The listing builds one solid part. Answer for the finished solid, in the listing's coordinates (mm). A direction names the side the tool comes from. Give positions to 0.01 mm unless a question says otherwise; leave off trailing zeros. Write each loop counter-clockwise with the first axis right and the second up, starting at its lowest first coordinate (ties: lowest second). Pieces come first, ordered by that corner, then holes.
```python
from build123d import *

# Parameters (mm, degrees)
SKETCH1_W             = 110
SKETCH1_H             = 64
SKETCH1_R             = 2.5
SKETCH1_W_2           = 40
SKETCH1_H_2           = 46
BOSS_EXTRUDE1_DEPTH   = 5
FILLET1_R             = 16
FILLET2_R             = 16
SKETCH2_W             = 50
SKETCH2_H             = 5
SKETCH2_W_2           = 20
BOSS_EXTRUDE2_DEPTH   = 46
BOSS_EXTRUDE3_START   = 51
SKETCH1_2_W           = 110
SKETCH1_2_H           = 64
SKETCH1_2_R           = 2.5
SKETCH1_2_W_2         = 40
SKETCH1_2_H_2         = 46
BOSS_EXTRUDE3_DEPTH   = 69
FILLET3_R             = 16
MIRROR2_START         = 120
MIRROR2_OUTLINE_R     = 2.5
MIRROR2_DEPTH         = 69
MIRROR2_START_2       = 235
MIRROR2_2_OUTLINE_R   = 2.5
MIRROR2_2_DEPTH       = 5
MIRROR2_START_3       = 189
MIRROR2_3_OUTLINE_W   = 20
MIRROR2_3_OUTLINE_H   = 5
MIRROR2_3_OUTLINE_W_2 = 50
MIRROR2_3_DEPTH       = 46


# Read off the part's stored shape, not the designer's step: Mirror2
with BuildPart() as part:
    # Sketch1 → Boss-Extrude1 (new body)
    with BuildSketch(Plane.XY):
        Rectangle(SKETCH1_W, SKETCH1_H)
        with Locations((39, 8)):
            Circle(SKETCH1_R, mode=Mode.SUBTRACT)
        with Locations((-39, 8)):
            Circle(SKETCH1_R, mode=Mode.SUBTRACT)
        Rectangle(SKETCH1_W_2, SKETCH1_H_2, mode=Mode.SUBTRACT)
    extrude(amount=BOSS_EXTRUDE1_DEPTH)

    # Fillet1
    fillet1_edges = [part.edges().sort_by_distance(p)[0] for p in [
        (55, -32, 2.5),
        (-55, -32, 2.5),
        (-55, 32, 2.5),
        (55, 32, 2.5),
    ]]
    fillet(fillet1_edges, radius=FILLET1_R)

    # Fillet2
    fillet2_edges = [part.edges().sort_by_distance(p)[0] for p in [
        (20, -23, 2.5),
        (20, 23, 2.5),
        (-20, 23, 2.5),
        (-20, -23, 2.5),
    ]]
    fillet(fillet2_edges, radius=FILLET2_R)

    # Sketch2 → Boss-Extrude2 (add)
    with BuildSketch(Plane.XY.offset(5)):
        with Locations((0, 29.5)):
            Rectangle(SKETCH2_W, SKETCH2_H)
        with Locations((0, -29.5)):
            Rectangle(SKETCH2_W_2, SKETCH2_H)
    extrude(amount=BOSS_EXTRUDE2_DEPTH)

    # Sketch1<2> → Boss-Extrude3 (add)
    with BuildSketch(Plane.XY.offset(BOSS_EXTRUDE3_START)):
        Rectangle(SKETCH1_2_W, SKETCH1_2_H)
        with Locations((39, 8)):
            Circle(SKETCH1_2_R, mode=Mode.SUBTRACT)
        with Locations((-39, 8)):
            Circle(SKETCH1_2_R, mode=Mode.SUBTRACT)
        Rectangle(SKETCH1_2_W_2, SKETCH1_2_H_2, mode=Mode.SUBTRACT)
    extrude(amount=BOSS_EXTRUDE3_DEPTH)

    # Fillet3
    fillet3_edges = [part.edges().sort_by_distance(p)[0] for p in [
        (55, 32, 85.5),
        (-55, 32, 85.5),
        (-55, -32, 85.5),
        (55, -32, 85.5),
        (-20, -23, 85.5),
        (20, -23, 85.5),
        (20, 23, 85.5),
        (-20, 23, 85.5),
    ]]
    fillet(fillet3_edges, radius=FILLET3_R)

    # Mirror2 outline → Mirror2 (add)
    with BuildSketch(Plane.XY.offset(MIRROR2_START)):
        with BuildLine():
            ThreePointArc((39, -32), (50.313708499, -27.313708499), (55, -16))
            Line((55, -16), (55, 16))
            ThreePointArc((55, 16), (50.313708499, 27.313708499), (39, 32))
            Line((39, 32), (-39, 32))
            ThreePointArc((-39, 32), (-50.313708499, 27.313708499), (-55, 16))
            Line((-55, 16), (-55, -16))
            ThreePointArc((-55, -16), (-50.313708499, -27.313708499), (-39, -32))
            Line((-39, -32), (39, -32))
        make_face()
        with Locations((-39, 8)):
            Circle(MIRROR2_OUTLINE_R, mode=Mode.SUBTRACT)
        with BuildLine():
            Line((20, 7), (20, -7))
            ThreePointArc((20, -7), (15.313708499, -18.313708499), (4, -23))
            Line((4, -23), (-4, -23))
            ThreePointArc((-4, -23), (-15.313708499, -18.313708499), (-20, -7))
            Line((-20, -7), (-20, 7))
            ThreePointArc((-20, 7), (-15.313708499, 18.313708499), (-4, 23))
            Line((-4, 23), (4, 23))
            ThreePointArc((4, 23), (15.313708499, 18.313708499), (20, 7))
        make_face(mode=Mode.SUBTRACT)
        with Locations((39, 8)):
            Circle(MIRROR2_OUTLINE_R, mode=Mode.SUBTRACT)
    extrude(amount=MIRROR2_DEPTH)



with BuildPart() as body_2:
    # Mirror2 2 outline → Mirror2 2 (new body)
    with BuildSketch(Plane.XY.offset(MIRROR2_START_2)):
        with BuildLine():
            ThreePointArc((39, -32), (50.313708499, -27.313708499), (55, -16))
            Line((55, -16), (55, 16))
            ThreePointArc((55, 16), (50.313708499, 27.313708499), (39, 32))
            Line((39, 32), (-39, 32))
            ThreePointArc((-39, 32), (-50.313708499, 27.313708499), (-55, 16))
            Line((-55, 16), (-55, -16))
            ThreePointArc((-55, -16), (-50.313708499, -27.313708499), (-39, -32))
            Line((-39, -32), (39, -32))
        make_face()
        with Locations((-39, 8)):
            Circle(MIRROR2_2_OUTLINE_R, mode=Mode.SUBTRACT)
        with BuildLine():
            Line((20, 7), (20, -7))
            ThreePointArc((20, -7), (15.313708499, -18.313708499), (4, -23))
            Line((4, -23), (-4, -23))
            ThreePointArc((-4, -23), (-15.313708499, -18.313708499), (-20, -7))
            Line((-20, -7), (-20, 7))
            ThreePointArc((-20, 7), (-15.313708499, 18.313708499), (-4, 23))
            Line((-4, 23), (4, 23))
            ThreePointArc((4, 23), (15.313708499, 18.313708499), (20, 7))
        make_face(mode=Mode.SUBTRACT)
        with Locations((39, 8)):
            Circle(MIRROR2_2_OUTLINE_R, mode=Mode.SUBTRACT)
    extrude(amount=MIRROR2_2_DEPTH)


with BuildPart() as part_1:
    add(part.part)

    add(body_2.part)  # Mirror2 3 merges body 2
    # Mirror2 3 outline → Mirror2 3 (add)
    with BuildSketch(Plane.XY.offset(MIRROR2_START_3)):
        with Locations((0, -29.5)):
            Rectangle(MIRROR2_3_OUTLINE_W, MIRROR2_3_OUTLINE_H)
        with Locations((0, 29.5)):
            Rectangle(MIRROR2_3_OUTLINE_W_2, MIRROR2_3_OUTLINE_H)
    extrude(amount=MIRROR2_3_DEPTH)


solid = part_1.part
```
Item 1: A cutting plane is placed at A-A, the plane x = -34. Give the vertices of the cut face in (y, z), plus the area to 3 significant figures.
Conclusion:
outline: (-32, 0) - (32, 0) - (32, 5) - (-32, 5) - close; (-32, 51) - (32, 51) - (32, 189) - (-32, 189) - close; (-32, 235) - (32, 235) - (32, 240) - (-32, 240) - close
area: 9,470 mm2
Item 2: A cutting plane is placed at C-C, the plane z = 32.5. Give the vertices of the cut face in (x, y), plus the area to 3 significant figures.
Conclusion:
outline: (-25, 27) - (25, 27) - (25, 32) - (-25, 32) - close; (-10, -32) - (10, -32) - (10, -27) - (-10, -27) - close
area: 350 mm2
Item 3: Each of these flat-tipped pins is pushed along its axis until it touches: P1, Ø5.5, axis at y = 29.5, z = 202.5, coming from the -X side; P2, Ø5.5, axis at y = -30.5, z = 207.5, coming from the +X side; P3, Ø8, axis at y = -21, z = 170, coming from the +X side; P4, Ø3, axis at x = 39, y = 8, coming from the +Z side. Where does it stop, or does it pass through?
Conclusion:
P1: stops at x = -25
P2: stops at x = 10
P3: stops at x = 54.97
P4: passes through
Item 4: Consider probe 1 along Z at (x, y) = (30.5, -8); probe 2 along Y at (x, z) = (-39, 1); probe 3 along X at (y, z) = (-4, 131.5). Determine where each line is inside the solid, lowest interval first.
Conclusion:
probe 1: z = 0 to 5, 51 to 189, 235 to 240
probe 2: y = -32 to 5.5, 10.5 to 32
probe 3: x = -55 to -20, 20 to 55
Item 5: Determine the mould class of faces 1 (the face through (-20, 0, 2)), 2 (the face through (24, 0, 5)), 3 (the face through (-50.437, 27.189, 2.535)) for opening direction X: pulls with the +X half, pulls with the -X half, needs draft (parallel to the pull), parting line crosses it, or undercut.
Conclusion:
face 1: undercut
face 2: needs draft
face 3: pulls with the -X half
Item 6: A cutting plane is placed at B-B, the plane z = 144.5. Give the vertices of the cut face in (x, y), plus the area to 3 significant figures.
Conclusion:
outline: (-55, -16) arc R16 ccw to (-39, -32) - (39, -32) arc R16 ccw to (55, -16) - (55, 16) arc R16 ccw to (39, 32) - (-39, 32) arc R16 ccw to (-55, 16) - close; hole circle Ø5 at (-39, 8); hole (-20, -7) arc R16 ccw to (-4, -23) - (4, -23) arc R16 ccw to (20, -7) - (20, 7) arc R16 ccw to (4, 23) - (-4, 23) arc R16 ccw to (-20, 7) - close; hole circle Ø5 at (39, 8)
area: 5,160 mm2
Item 7: Which of the six approach directions +Z, -Z, +X, -X, +Y, -Y give full straight-line access (tool end or side, diameter ignored) to faces 4 (the face through (20, 0, 2)), 5 (the face through (-50.437, -27.189, 2.535)), 6 (the face through (10, -30, 28))?
Conclusion:
face 4: +Z, -Z
face 5: +Z, -Z, -X, -Y
face 6: +X, -Y
Item 8: A cutting plane is placed at D-D, the plane y = -12. Give the vertices of the cut face in (x, z), plus the area to 3 significant figures.
Conclusion:
outline: (-55, 0) - (-19.2, 0) - (-19.2, 5) - (-55, 5) - close; (-55, 51) - (-19.2, 51) - (-19.2, 189) - (-55, 189) - close; (-55, 235) - (-19.2, 235) - (-19.2, 240) - (-55, 240) - close; (19.2, 0) - (55, 0) - (55, 5) - (19.2, 5) - close; (19.2, 51) - (55, 51) - (55, 189) - (19.2, 189) - close; (19.2, 235) - (55, 235) - (55, 240) - (19.2, 240) - close
area: 10,600 mm2
